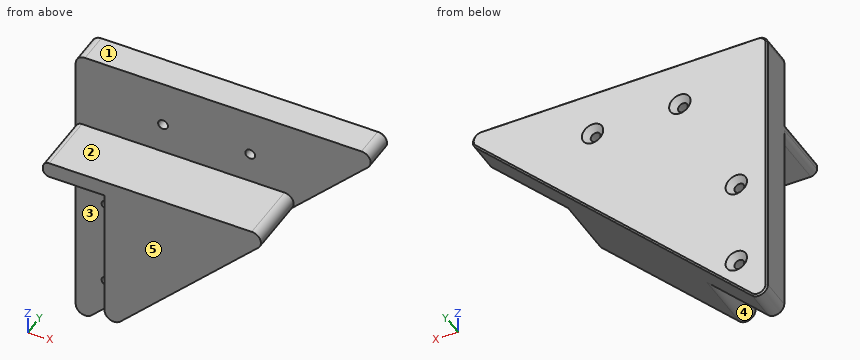
from build123d import *

# Parameters (mm, degrees)
SKETCH1_R                                            = 1
MAIN_BODY_DEPTH                                      = 10.5
PROFILE_STOPS_DEPTH                                  = 20
CSK_FOR_M3_HEX_SOCKET_COUNTERSUNK_HEAD_S_D           = 3.2
CSK_FOR_M3_HEX_SOCKET_COUNTERSUNK_HEAD_S_DEPTH       = 30.5
CSK_FOR_M3_HEX_SOCKET_COUNTERSUNK_HEAD_S_CSINK_D     = 6.94
CSK_FOR_M3_HEX_SOCKET_COUNTERSUNK_HEAD_S_CSINK_ANGLE = 90
FILLET1_R                                            = 3
FILLET3_R                                            = 2
CHAMFER1_SIZE                                        = 0.5


with BuildPart() as part:
    # Sketch1 → Main Body (new body)
    with BuildSketch(Plane(origin=(0, 0, 0), x_dir=(1, 0, 0), z_dir=(0, 1, 0))):
        Polygon((-48, -6.5), (52, -6.5), (-48, 93.5), align=None)
        with Locations((-19.666666667, 8.5)):
            Circle(SKETCH1_R, mode=Mode.SUBTRACT)
        with Locations((8.666666667, 8.5)):
            Circle(SKETCH1_R, mode=Mode.SUBTRACT)
        with Locations((-38, 45.516187598)):
            Circle(SKETCH1_R, mode=Mode.SUBTRACT)
        with Locations((-38, 73.849520931)):
            Circle(SKETCH1_R, mode=Mode.SUBTRACT)
    extrude(amount=MAIN_BODY_DEPTH)

    # Sketch1_3 → Profile Stops (add)
    with BuildSketch(Plane(origin=(0, 0, 0), x_dir=(1, 0, 0), z_dir=(0, 1, 0))):
        Polygon((-48, 23.5), (-48, 18.5), (27, 18.5), (-28, 73.5), (-28, 23.5), (-41, 23.5), align=None)
    extrude(amount=-PROFILE_STOPS_DEPTH)

    # CSK for M3 Hex Socket Countersunk Head S
    with Locations(Plane(origin=(-38, 10.5, -73.849520931), x_dir=(0, 0, 1), z_dir=(0, 1, 0))):
        with Locations((0, 0), (28.333333333, 0), (65.349520931, 46.666666667), (65.349520931, 18.333333333)):
            CounterSinkHole(CSK_FOR_M3_HEX_SOCKET_COUNTERSUNK_HEAD_S_D / 2, CSK_FOR_M3_HEX_SOCKET_COUNTERSUNK_HEAD_S_CSINK_D / 2, depth=CSK_FOR_M3_HEX_SOCKET_COUNTERSUNK_HEAD_S_DEPTH, counter_sink_angle=CSK_FOR_M3_HEX_SOCKET_COUNTERSUNK_HEAD_S_CSINK_ANGLE)

    # Fillet1
    fillet1_edges = [part.edges().sort_by_distance(p)[0] for p in [
        (-48, 5.25, 6.5),
        (52, 5.25, 6.5),
        (-28, -10, -73.5),
        (27, -10, -18.5),
        (-48, 5.25, -93.5),
    ]]
    fillet(fillet1_edges, radius=FILLET1_R)

    # Fillet3
    fillet3_edges = [part.edges().sort_by_distance(p)[0] for p in [
        (-48, -10, -23.5),
        (-48, -10, -18.5),
    ]]
    fillet(fillet3_edges, radius=FILLET3_R)

    # Chamfer1
    chamfer1_edges = [part.edges().sort_by_distance(p)[0] for p in [
        (-48, 10.5, -41.378679656),
        (2, 10.5, -43.5),
        (-47.121320344, 10.5, 5.621320344),
        (47.52899791, 10.5, 4.648050297),
        (-0.121320344, 10.5, 6.5),
        (-46.148050297, 10.5, -89.02899791),
    ]]
    chamfer(chamfer1_edges, length=CHAMFER1_SIZE)


solid = part.part
Can you work these out from the model? Positions are in its coordinate system, mm. Face numbers are marked on the shaded views. A direction names the side the tool comes from. Coordinates: 2 decimals unless noted, no trailing zeros. Order: outer loops, then holes, each group sorted by start corner. A loop starts at its lowest first (then second) coordinate and runs counter-clockwise, first axis right, second up. Notation, with made-up numbers: M 45.25,74 L 89.25,74 A8 cw 89.25,78 Z; hole C 19,71.25 d9. An arc over 180 degrees is marked long. Answer as CSV lines item,"result".
(1) Suppose I cut it at C-C on y = 5.5. Please give me the cut outline in (x, z), plus the area to 3 significant figures.
Geometry check:
outline,"M -48,-86.26 A3 ccw -42.88,-88.38 L 46.88,1.38 A3 ccw 44.76,6.5 L -45,6.5 A3 ccw -48,3.5 Z; hole C -38,-73.85 d3.2; hole C -38,-45.52 d3.2; hole C -19.67,-8.5 d3.2; hole C 8.67,-8.5 d3.2"
area,"4,940 mm^2"
(2) Suppose I cut it at A-A on z = -8.5. Please give me the cut outline in (x, y).
Geometry check:
outline,"M -48,0 L -21.27,0 L -21.27,8.63 L -23.14,10.5 L -47.5,10.5 L -48,10 Z; M -18.07,0 L 7.07,0 L 7.07,8.63 L 5.2,10.5 L -16.2,10.5 L -18.07,8.63 Z; M 10.27,0 L 37,0 L 37,10 L 36.29,10.5 L 12.14,10.5 L 10.27,8.63 Z"
(3) Suppose I cut it at B-B on x = -38. Please give me the cut outline in (y, z), plus the area to 3 significant figures.
Geometry check:
outline,"M -20,-23.5 L 0,-23.5 L 0,-43.92 L 8.63,-43.92 L 10.5,-42.05 L 10.5,6 L 10,6.5 L 0,6.5 L 0,-18.5 L -20,-18.5 Z; M 0,-83.5 L 10,-83.5 L 10.5,-82.79 L 10.5,-77.32 L 8.63,-75.45 L 0,-75.45 Z; M 0,-72.25 L 8.63,-72.25 L 10.5,-70.38 L 10.5,-48.99 L 8.63,-47.12 L 0,-47.12 Z"
area,"971 mm^2"
(4) I'm going to push flat-ended pins straight in: pin 1 (5 mm diameter, centred on x = 3.5, y = -10.5, fed in from +Z); pin 2 (7.5 mm diameter, centred on x = -39, z = -44.5, fed in from -Y); pin 3 (5 mm diameter, centred on x = -38, z = -45.52, fed in from +Y). Where does each tip first touch, or does it pass through?
Geometry check:
pin 1,"z = -18.5"
pin 2,"y = 0"
pin 3,"y = 9.53"
(5) Please list where these lines run through material, in increasing order: L1, parallel to X at y = 5.75, z = -8.5; L2, parallel to Y at x = 3.5, z = -16; L3, parallel to Z at x = -38, y = 7.
Geometry check:
L1,"-48 to -21.27, -18.07 to 7.07, 10.27 to 37"
L2,"0 to 10.5"
L3,"-83.5 to -75.45, -72.25 to -47.12, -43.92 to 6.5"
(6) Suppose I cut it at D-D on x = -13.5. Please give me the cut outline in (y, z).
Geometry check:
outline,"M -20,-59 L 10,-59 L 10.5,-58.29 L 10.5,6 L 10,6.5 L 0,6.5 L 0,-18.5 L -20,-18.5 Z"
(7) On a 3-axis mill with a long thin cutter (end or side, diameter ignored), from which of +Z, -Z, +X, -X, +Y, -Y can I reach the whole of each face in a straight line? I mean the marked faces 1, 2, 3, 4 and 5. Say none if no direction works.
Geometry check:
face 1,"+Z, +X, -X, +Y, -Y"
face 2,"+Z, +X, -X, -Y"
face 3,"-Z, -X, -Y"
face 4,"-Z, -Y"
face 5,"+Z, -Z, +X, -X, -Y"
